Check sheet for the modelled part. Datum: model origin and axes. Units: mm. A direction names the side the tool comes from. Round coordinates to 2 decimals unless told otherwise and drop trailing zeros. Write each loop counter-clockwise with the first axis right and the second up, starting at its lowest first coordinate (ties: lowest second). Pieces come first, ordered by that corner, then holes.
Item 1: Cross-section at C-C on x = -2.5. Enter the section's corners in (y, z).
Item 2: Cross-section at D-D on z = 4. Enter the section's corners in (x, y), plus the area to 3 significant figures.
Item 3: Tool access check on faces 5 (the flat face through (-2, 5, 4)), 6 (the flat face through (-8, 7, 10)), 7 (the flat face through (-9, 16, 10)), 8 (the flat face through (-1, 20.3, 10)). Record the directions out of +Z, -Z, +X, -X, +Y, -Y that give a thin tool (end or side, any length) a straight path to the whole face; none if there is none.
Item 4: Cross-section at A-A on z = 18.75. Enter the section's corners in (x, y).
Item 5: Release check for a two-part mould opening along Z. For faces 1 (the cylindrical face through (-3.7, 2.5, 17.6)), 2 (the cylindrical face through (-10.502, 7.166, 10.14)), 3 (the flat face through (-6, 12, 0)), 4 (the flat face through (-6, 12, 20)) record: +Z half, -Z half, draft (parallel to the pull), parting line (faces both ways), or undercut.
Item 6: Cross-section at B-B on y = 2.25. Enter the section's corners in (x, z), plus the area to 3 significant figures.
Item 7: Material ranges on line 1 (X direction, y = 3.05, z = 4); line 2 (Z direction, x = -3.75, y = 3.75); line 3 (X direction, y = 2, z = 1), recorded low to high.
Item 8: Go/stop test with flat-tipped pins: pin 1 Ø3 at (y, z) = (4, 13) entering from -X; pin 2 Ø8 at (y, z) = (19.5, 16.5) entering from +X; pin 3 Ø0.9 at (y, z) = (22.5, 12) entering from +X; pin 4 Ø2.5 at (x, z) = (-2.5, 4) entering from -Y. Record where each tip stops, or that it passes through.
from build123d import *

# Parameters (mm, degrees)
BOSS_EXTRU_1_DEPTH      = 20
CONG_1_R                = 1
ESQUISSE3_R             = 2
ENL_V_MAT_EXTRU_1_DEPTH = 5


with BuildPart() as part:
    # Esquisse1 → Boss.-Extru.1 (new body)
    with BuildSketch(Plane.XY):
        Polygon((-2, 23.3), (-5, 23.3), (-5, 16), (-14.6, 16), (-10.6, 7), (-5, 7), (-5, 0), (0, 0), (0, 20.3), (-2, 20.3), align=None)
    extrude(amount=BOSS_EXTRU_1_DEPTH)

    # Congé1
    cong_1_edges = [part.edges().sort_by_distance(p)[0] for p in [
        (-10.6, 7, 10),
        (-14.6, 16, 10),
        (-5, 23.3, 10),
    ]]
    fillet(cong_1_edges, radius=CONG_1_R)

    # Esquisse3 → Enlèv. mat.-Extru.1 (cut)
    with BuildSketch(Plane.XZ):
        with Locations(Location((-2.5, 4, 0), (0, 0, 270))):
            Circle(ESQUISSE3_R)
        with Locations(Location((-2.5, 16, 0), (0, 0, 270))):
            Circle(ESQUISSE3_R)
    extrude(amount=-ENL_V_MAT_EXTRU_1_DEPTH, mode=Mode.SUBTRACT)


solid = part.part
Response values:
1. outline: (0, 0) - (23.3, 0) - (23.3, 20) - (0, 20) - (0, 18) - (5, 18) - (5, 14) - (0, 14) - (0, 6) - (5, 6) - (5, 2) - (0, 2) - close
2. outline: (-13.98, 14.59) - (-10.86, 7.59) arc R1 ccw to (-9.95, 7) - (-5, 7) - (-5, 0) - (-4.5, 0) - (-4.5, 5) - (-0.5, 5) - (-0.5, 0) - (0, 0) - (0, 20.3) - (-2, 20.3) - (-2, 23.3) - (-4, 23.3) arc R1 ccw to (-5, 22.3) - (-5, 16) - (-13.06, 16) arc R1 ccw to start
2. area: 158 mm2
3. face 5: -Y
3. face 6: +Z, -Z, -X, -Y
3. face 7: +Z, -Z, -X, +Y
3. face 8: +Z, -Z, +X, +Y
4. outline: (-13.98, 14.59) - (-10.86, 7.59) arc R1 ccw to (-9.95, 7) - (-5, 7) - (-5, 0) - (0, 0) - (0, 20.3) - (-2, 20.3) - (-2, 23.3) - (-4, 23.3) arc R1 ccw to (-5, 22.3) - (-5, 16) - (-13.06, 16) arc R1 ccw to start
5. face 1: undercut
5. face 2: draft
5. face 3: -Z half
5. face 4: +Z half
6. outline: (-5, 0) - (0, 0) - (0, 20) - (-5, 20) - close; hole circle Ø4 at (-2.5, 4); hole circle Ø4 at (-2.5, 16)
6. area: 74.9 mm2
7. line 1: x = -5 to -4.5, -0.5 to 0
7. line 2: z = 0 to 2.44, 5.56 to 14.44, 17.56 to 20
7. line 3: x = -5 to 0
8. pin 1: stops at x = -5
8. pin 2: stops at x = 0
8. pin 3: stops at x = -2
8. pin 4: stops at y = 5
